Design review of the part built by this model. Coordinates are the model's own, in mm. Coordinates: 2 decimals unless noted, no trailing zeros. Loops run counter-clockwise (first coordinate to the right, second up) from the corner with the lowest first, then second, coordinate; pieces in that order, holes last. Notation, with made-up numbers: M -2.5,80.25 L 25.5,80.25 A11 ccw 25.5,86.25 Z; hole C 21,-8.5 d8. An arc over 180 degrees is marked long. Write item = value, one per line. Start each with the question number.
```python
from build123d import *

# Parameters (mm, degrees)
ESQUISSEREF_R    = 20
ESQUISSEREF_R_2  = 5
ESQUISSEREF_R_3  = 25
EXTRUSION1_DEPTH = 8


with BuildPart() as part:
    # EsquisseRef → Extrusion1 (new body)
    with BuildSketch(Plane.XY):
        Polygon((-693, 248), (245, 248), (245, 165), (191, 165), (191, 145), (245, 145), (245, -60), (-693, -60), align=None)
        Circle(ESQUISSEREF_R, mode=Mode.SUBTRACT)
        with Locations((-621, 197.5)):
            Circle(ESQUISSEREF_R_2, mode=Mode.SUBTRACT)
        with Locations((-566, 197.5)):
            Circle(ESQUISSEREF_R_2, mode=Mode.SUBTRACT)
        with Locations((-566, 112.5)):
            Circle(ESQUISSEREF_R_2, mode=Mode.SUBTRACT)
        with Locations((-621, 112.5)):
            Circle(ESQUISSEREF_R_2, mode=Mode.SUBTRACT)
        with Locations((142, 0)):
            Circle(ESQUISSEREF_R_3, mode=Mode.SUBTRACT)
    extrude(amount=-EXTRUSION1_DEPTH)


solid = part.part
```
(1) To check wall thickness, follow L1, parallel to Y at x = -566, z = -2.75; L2, parallel to Y at x = 142, z = -1.75; L3, parallel to Y at x = 0, z = -3. State the ranges of each line that lie inside material, in increasing order.
(2) Take a section at A-A (x = 0). State the section outline as (y, z) points, plus the area to 3 significant figures.
(3) Mouldability with a two-part tool opening along X and no side actions: class faces 1 (the flat face through (-217, 96, -8)), 2 (the cylindrical face through (-4.336, -19.524, -3.944)) as +X half, -X half, draft (parallel to the pull), parting line (faces both ways), or undercut.
(4) Take a section at C-C (z = -2.25). State the section outline as (x, y) points.
(5) Take a section at B-B (y = 0). State the section outline as (x, z) points.
Results list:
q1.L1 = -60 to 107.5, 117.5 to 192.5, 202.5 to 248
q1.L2 = -60 to -25, 25 to 248
q1.L3 = -60 to -20, 20 to 248
q2.outline = M -60,-8 L -20,-8 L -20,0 L -60,0 Z; M 20,-8 L 248,-8 L 248,0 L 20,0 Z
q2.area = 2,140 mm^2
q3.face_1 = draft
q3.face_2 = undercut
q4.outline = M -693,-60 L 245,-60 L 245,145 L 191,145 L 191,165 L 245,165 L 245,248 L -693,248 Z; hole C -621,112.5 d10; hole C -621,197.5 d10; hole C -566,112.5 d10; hole C -566,197.5 d10; hole C 0,0 d40; hole C 142,0 d50
q5.outline = M -693,-8 L -20,-8 L -20,0 L -693,0 Z; M 20,-8 L 117,-8 L 117,0 L 20,0 Z; M 167,-8 L 245,-8 L 245,0 L 167,0 Z
